Solid Edge part; units mm, degrees
sketch "Sketch1" plane through (0, 0, 0) normal (0, -1, 0) x (1, 0, 0)
  line L0 (8, 6) -> (-8, 6)
  line L1 (-8, 6) -> (-8, -6)
  line L2 (-8, -6) -> (8, -6)
  line L3 (8, -6) -> (8, 6)
extrude "Protrusion1" add sketch "Sketch1" against normal blind 22
sketch "Sketch2" plane through (0, 0, 0) normal (0, -1, 0) x (1, 0, 0)
  line L0 (6, 4.25) -> (-6.5, 4.25)
  line L1 (-6.5, 4.25) -> (-6.5, -4.25)
  line L2 (-6.5, -4.25) -> (6, -4.25)
  line L3 (6, -4.25) -> (6, 4.25)
extrude "Cutout1" cut sketch "Sketch2" against normal blind 20
sketch "Sketch3" plane through (0, 20, 0) normal (0, -1, 0) x (1, 0, 0)
  line L0 (6, -3) -> (2, -3)
  line L1 (2, -3) -> (2, -4)
  line L2 (2, -4) -> (6, -4)
  line L3 (6, -4) -> (6, -3)
  line L4 (6, 3) -> (2.0028, 3)
  line L5 (2.0028, 3) -> (2.0028, 4.25)
  line L6 (2.0028, 4.25) -> (6, 4.25)
  line L7 (6, 4.25) -> (6, 3)
extrude "LockSideProtrusion" add sketch "Sketch3" along normal blind 19
sketch "Sketch4" plane through (0, 20, 0) normal (0, -1, 0) x (1, 0, 0)
  line L0 (6, 3) -> (6, -3)
  line L1 (6, -3) -> (2.0028, -3)
  line L2 (2.0028, -3) -> (2.0028, 3)
  line L3 (2.0028, 3) -> (6, 3)
extrude "LockBaseProtrusion" add sketch "Sketch4" along normal blind 2
sketch "Sketch5" plane through (4.0014, 18, 0) normal (0, -1, 0) x (1, 0, 0)
  line L0 (-0.0014, 2.48) -> (-0.0014, -2.48)
  line L1 (-0.0014, -2.48) -> (-2.0014, -2.48)
  line L2 (-2.0014, -2.48) -> (-2.0014, 2.48)
  line L3 (-2.0014, 2.48) -> (-0.0014, 2.48)
extrude "LockProtrusion" add sketch "Sketch5" along normal blind 18.07
sketch "Sketch6" plane through (3, -0.07, 0) normal (0, -1, 0) x (1, 0, 0)
  line L0 (-1, -4.18) -> (-1, 3.68)
  line L1 (-1, 3.68) -> (1, 3.68)
  line L2 (1, 3.68) -> (1, -4.18)
  line L3 (1, -4.18) -> (-1, -4.18)
extrude "LockHeadMainProtrusion" add sketch "Sketch6" along normal blind 3
sketch "Sketch7" plane through (3, -0.07, 0) normal (0, -1, 0) x (1, 0, 0)
  line L0 (-3.4, 3.68) -> (-1, 1.28)
  line L1 (-1, 1.28) -> (-1, 3.68)
  line L2 (-1, 3.68) -> (-3.4, 3.68)
  line L3 (-3.4, -4.18) -> (-1, -1.78)
  line L4 (-1, -1.78) -> (-1, -4.18)
  line L5 (-1, -4.18) -> (-3.4, -4.18)
extrude "LockHeadTriangleProtrusion" add sketch "Sketch7" along normal blind 3
sketch "Sketch8" plane through (1.8, -1.57, -4.18) normal (0, 0, -1) x (1, 0, 0)
  line L0 (-2.2, 1.5) -> (0.2, 1.5)
  line L1 (0.2, 1.5) -> (-2.2, -1.5)
  line L2 (-2.2, -1.5) -> (-2.2, 1.5)
extrude "LockHeadTriangleCut" cut sketch "Sketch8" against normal blind 8.6519
sketch "Sketch9" plane through (4, 7.465, 0) normal (1, 0, 0) x (0, 0, 1)
  line L0 (-4.18, 10.535) -> (3.93, 10.535)
  line L1 (3.93, 10.535) -> (3.93, 8.535)
  line L2 (3.93, 8.535) -> (-4.18, 8.535)
  line L3 (-4.18, 8.535) -> (-4.18, 10.535)
extrude "FlapBaseProtrusion" add sketch "Sketch9" along normal blind 4
sketch "Sketch10" plane through (5, -3.07, 0) normal (0, -1, 0) x (1, 0, 0)
  line L0 (3, 3.93) -> (1, 3.93)
  line L1 (1, 3.93) -> (1, -3.93)
  line L2 (1, -3.93) -> (3, -3.93)
  line L3 (3, -3.93) -> (3, 3.93)
extrude "FlapHandleProtrusion" add sketch "Sketch10" along normal blind 2
fillet "SlotInnerRound" radius 1 3 edges at (-0.25, 0, 4.25) (-6.5, 0, 0) (-0.25, 0, -4.25)
fillet "FlapRound" radius 1 3 edges at (6, -5.07, 0) (8, -5.07, 0) (8, -1.07, -0.125)
sketch "Sketch11" plane through (4, -3.07, 0) normal (0, -1, 0) x (-1, 0, 0)
  line L0 (-1.6753, 0.0864) -> (1.042, 1.2263)
  line L1 (1.042, 1.2263) -> (1.042, -1.1917)
  line L2 (1.042, -1.1917) -> (-1.6753, 0.0864)
extrude "MarkCut" cut sketch "Sketch11" against normal blind 0.8
hole "PushHole" at (-2.0513, 20, 0) direction (0, 1, 0) diameter 4 end through all
fillet "LockTriangleRound" radius 1 2 edges at (2, -1.57, 1.28) (2, -1.57, -1.78)
sketch "Sketch12" plane through (1.8, -1.57, 3.68) normal (0, 0, 1) x (1, 0, 0)
  line L0 (2.2, 0.725) -> (2.2, 0.3676)
  line L1 (2.2, 0.3676) -> (2.2, -1.5)
  line L2 (2.2, -1.5) -> (0.2, -1.5)
  line L3 (0.2, -1.5) -> (-2.2, 1.5)
  line L4 (-2.2, 1.5) -> (2.2, 1.5)
  line L5 (2.2, 1.5) -> (2.2, 0.725)
extrude "Protrusion2" add sketch "Sketch12" along normal blind 0.2509
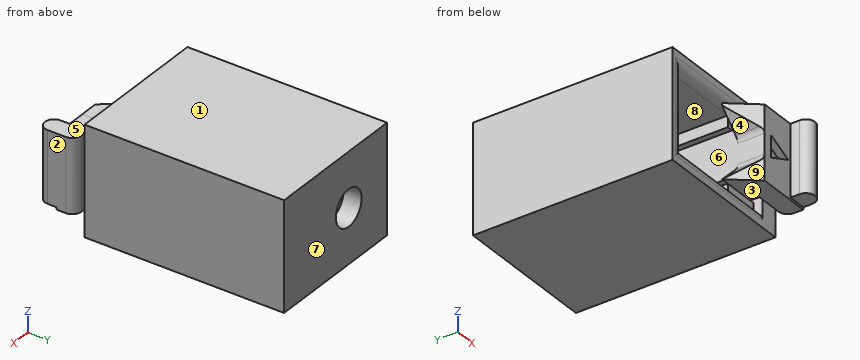
Geometry check sheet. Reference: the model listing, model coordinates, mm. Face numbers are marked on the shaded views. A direction names the side the tool comes from. Give positions to 0.01 mm unless a question says otherwise; leave off trailing zeros. Order: outer loops, then holes, each group sorted by start corner. A loop starts at its lowest first (then second) coordinate and runs counter-clockwise, first axis right, second up. Notation, with made-up numbers: (20.25, -23) - (36.25, -23) arc R31 ccw to (36.25, 15) - close; hole circle Ø10 at (-19, 31.25). An arc over 180 degrees is marked (long way). Answer in a Markdown table with one row per item. Add a question column.
Q1. Cross-section at D-D, the plane x = -3.5. Enter the section's corners in (y, z), then the cut area to 3 significant figures.
Q2. Gauge pin test, flat ends, axial feed: pin 1 (1.5 mm diameter, centred on x = 1, z = 3.5, fed in from -Y); pin 2 (4.5 mm diameter, centred on x = 7, y = -2.5, fed in from +Z); pin 3 (0.5 mm diameter, centred on x = 3.5, z = -3.5, fed in from -Y). Record the tip position at first contact, or that the pin passes through.
Q3. Cross-section at C-C, the plane x = -5.5. Enter the section's corners in (y, z), then the cut area to 3 significant figures.
Q4. Cross-section at B-B, the plane y = 1.5. Enter the section's corners in (x, z).
Q5. Mould release check, pull along Y, two halves, no side actions. Record for the marked faces 6, 7, 8 and 9: pulls with the +Y half, pulls with the -Y half, needs draft (parallel to the pull), parting line crosses it, or undercut.
Q6. Material ranges on probe 1 along Z at (x, y) = (2.75, 10); probe 2 along X at (y, z) = (21.15, 0); probe 3 along Z at (x, y) = (-5.25, 3), recorded low to high. Write a range as from..to.
Q7. Tool access check on the marked faces 1, 2, 3, 4 and 5. Record the directions out of +Z, -Z, +X, -X, +Y, -Y that give a thin tool (end or side, any length) a straight path to the whole face; none if there is none.
Check values:
| question | item | result |
|---|---|---|
| 1 | outline | (0, -6) - (22, -6) - (22, -1.38) - (20, -1.38) - (20, -4.25) - (1, -4.25) arc R1 ccw to (0, -5.25) - close; (0, 5.25) arc R1 ccw to (1, 4.25) - (20, 4.25) - (20, 1.38) - (22, 1.38) - (22, 6) - (0, 6) - close |
| 1 | area | 88.1 mm^2 |
| 2 | pin 1 | stops at y = -2.76 |
| 2 | pin 2 | stops at z = 3.93 |
| 2 | pin 3 | stops at y = -3.07 |
| 3 | outline | (0, -6) - (22, -6) - (22, 6) - (0, 6) - (0, 5.25) arc R1 ccw to (1, 4.25) - (20, 4.25) - (20, -4.25) - (1, -4.25) arc R1 ccw to (0, -5.25) - close |
| 3 | area | 93.6 mm^2 |
| 4 | outline | (-8, -6) - (8, -6) - (8, 6) - (-8, 6) - close; (2, -2.48) - (4, -2.48) - (4, 2.48) - (2, 2.48) - close; hole (-6.5, -4.25) - (6, -4.25) - (6, -4) - (2, -4) - (2, -3) - (6, -3) - (6, 3) - (2, 3) - (2, 4.25) - (-6.5, 4.25) - close |
| 5 | face 6 | undercut |
| 5 | face 7 | pulls with the +Y half |
| 5 | face 8 | needs draft |
| 5 | face 9 | pulls with the -Y half |
| 6 | probe 1 | z = -6..-4.25, -4..-3, -2.48..2.48, 3..6 |
| 6 | probe 2 | x = -8..-4.05, -0.05..8 |
| 6 | probe 3 | z = -6..-4.25, 4.25..6 |
| 7 | face 1 | +Z, +X, -X, +Y, -Y |
| 7 | face 2 | +Z, -Z, +X, +Y, -Y |
| 7 | face 3 | -Z, +X, -X, -Y |
| 7 | face 4 | -X, -Y |
| 7 | face 5 | +Z, +X, -X, -Y |
